Source: CAD feature listing. Evaluate the final solid. Frame: model axes, mm. Coordinates: 2 decimals unless noted, no trailing zeros. Loops run counter-clockwise (first coordinate to the right, second up) from the corner with the lowest first, then second, coordinate; pieces in that order, holes last.
```python
from build123d import *

# Parameters (mm, degrees)
SKETCH_1_R          = 2
SKETCH_1_R_2        = 11
EXTRUDE_1_DEPTH     = 4
SKETCH_3_W          = 126
SKETCH_3_H          = 2.7
CUT_EXTRUDE_1_DEPTH = 10


with BuildPart() as part:
    # 草图1 → 凸台-拉伸1 (new body)
    with BuildSketch(Plane.XY):
        Polygon((145, 46.5), (149, 46.5), (149, 45.15), (151.6, 45.15), (151.6, 46.5), (153.6, 46.5), (153.6, 49.5), (151.6, 49.5), (151.6, 50.85), (149, 50.85), (149, 49.5), (145, 49.5), (145, 59), (141, 59), (141, 67), (145, 67), (145, 76.5), (149, 76.5), (149, 75.15), (151.6, 75.15), (151.6, 76.5), (153.6, 76.5), (153.6, 79.5), (151.6, 79.5), (151.6, 80.85), (149, 80.85), (149, 79.5), (145, 79.5), (145, 89), (141, 89), (141, 97), (145, 97), (145, 106.5), (149, 106.5), (149, 105.15), (151.6, 105.15), (151.6, 106.5), (153.6, 106.5), (153.6, 109.5), (151.6, 109.5), (151.6, 110.85), (149, 110.85), (149, 109.5), (145, 109.5), (145, 123), (271, 123), (271, 109.5), (267, 109.5), (267, 110.85), (264.4, 110.85), (264.4, 109.5), (262.4, 109.5), (262.4, 106.5), (264.4, 106.5), (264.4, 105.15), (267, 105.15), (267, 106.5), (271, 106.5), (271, 97), (275, 97), (275, 89), (271, 89), (271, 79.5), (267, 79.5), (267, 80.85), (264.4, 80.85), (264.4, 79.5), (262.4, 79.5), (262.4, 76.5), (264.4, 76.5), (264.4, 75.15), (267, 75.15), (267, 76.5), (271, 76.5), (271, 67), (275, 67), (275, 59), (271, 59), (271, 49.5), (267, 49.5), (267, 50.85), (264.4, 50.85), (264.4, 49.5), (262.4, 49.5), (262.4, 46.5), (264.4, 46.5), (264.4, 45.15), (267, 45.15), (267, 46.5), (271, 46.5), (271, 37), (275, 37), (275, 29), (271, 29), (271, 19.5), (267, 19.5), (267, 20.85), (264.4, 20.85), (264.4, 19.5), (262.4, 19.5), (262.4, 16.5), (264.4, 16.5), (264.4, 15.15), (267, 15.15), (267, 16.5), (271, 16.5), (271, 7), (275, 7), (275, -1), (271, -1), (271, -10.5), (267, -10.5), (267, -9.15), (264.4, -9.15), (264.4, -10.5), (262.4, -10.5), (262.4, -13.5), (264.4, -13.5), (264.4, -14.85), (267, -14.85), (267, -13.5), (271, -13.5), (271, -27), (271, -34), (145, -34), (145, -27), (145, -13.5), (149, -13.5), (149, -14.85), (151.6, -14.85), (151.6, -13.5), (153.6, -13.5), (153.6, -10.5), (151.6, -10.5), (151.6, -9.15), (149, -9.15), (149, -10.5), (145, -10.5), (145, -1), (141, -1), (141, 7), (145, 7), (145, 16.5), (149, 16.5), (149, 15.15), (151.6, 15.15), (151.6, 16.5), (153.6, 16.5), (153.6, 19.5), (151.6, 19.5), (151.6, 20.85), (149, 20.85), (149, 19.5), (145, 19.5), (145, 29), (141, 29), (141, 37), (145, 37), align=None)
        with Locations((208, 29)):
            Circle(SKETCH_1_R, mode=Mode.SUBTRACT)
        with Locations((208, 48)):
            Circle(SKETCH_1_R_2, mode=Mode.SUBTRACT)
        with Locations((188, 8)):
            Circle(SKETCH_1_R, mode=Mode.SUBTRACT)
        with Locations((228, 8)):
            Circle(SKETCH_1_R, mode=Mode.SUBTRACT)
        with Locations((228, 88)):
            Circle(SKETCH_1_R, mode=Mode.SUBTRACT)
        with Locations((188, 88)):
            Circle(SKETCH_1_R, mode=Mode.SUBTRACT)
        with Locations((208, 8)):
            Circle(SKETCH_1_R, mode=Mode.SUBTRACT)
        with Locations((194.564971157, 34.564971157)):
            Circle(SKETCH_1_R, mode=Mode.SUBTRACT)
        with Locations((189, 48)):
            Circle(SKETCH_1_R, mode=Mode.SUBTRACT)
        with Locations((194.564971157, 61.435028843)):
            Circle(SKETCH_1_R, mode=Mode.SUBTRACT)
        with Locations((208, 67)):
            Circle(SKETCH_1_R, mode=Mode.SUBTRACT)
        with Locations((221.435028843, 61.435028843)):
            Circle(SKETCH_1_R, mode=Mode.SUBTRACT)
        with Locations((227, 48)):
            Circle(SKETCH_1_R, mode=Mode.SUBTRACT)
        with Locations((221.435028843, 34.564971157)):
            Circle(SKETCH_1_R, mode=Mode.SUBTRACT)
    extrude(amount=EXTRUDE_1_DEPTH)

    # 草图3 → 切除-拉伸1 (cut)
    with BuildSketch(Plane.XY.offset(4)):
        with Locations((208, 121.65)):
            Rectangle(SKETCH_3_W, SKETCH_3_H)
    extrude(amount=-CUT_EXTRUDE_1_DEPTH, mode=Mode.SUBTRACT)


solid = part.part
```
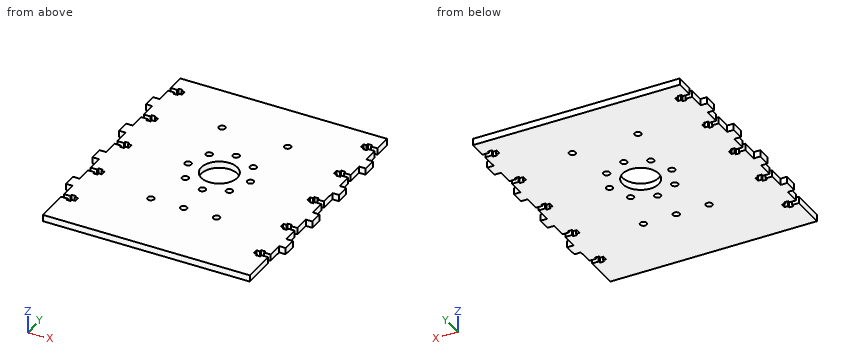
Q1. Material intervals for line 1 along Y through (x, z) = (149.5, 2); line 2 along Y through (x, z) = (269, 3.35); line 3 along Y through (x, z) = (208, 1.65), sorted ascending.
Q2. Section query B-B on z = 2.55. Count the separate pieces of the cut face and the enclosed holes in it, then the cut area to 3 significant figures.
Q3. First-contact query: pin 1 Ø1.1 at (y, z) = (-14, 2.5) entering from +X; pin 2 Ø1.1 at (y, z) = (105.5, 2.5) entering from -X; pin 3 Ø3 at (x, y) = (221.44, 34.56) entering from +Z; pin 4 Ø1.5 at (y, z) = (107.5, 2) entering from -X. Flat tips, straight axial feed; report the tip coordinate or a pass-through.
Q4. Section query A-A on x = 208. Return the cut outline in (y, z), then the cut area to 3 significant figures.
Resolved:
1. line 1: y = -34 to -14.85, -9.15 to 15.15, 20.85 to 45.15, 50.85 to 75.15, 80.85 to 105.15, 110.85 to 120.3
1. line 2: y = -34 to -13.5, -10.5 to 16.5, 19.5 to 46.5, 49.5 to 76.5, 79.5 to 106.5, 109.5 to 120.3
1. line 3: y = -34 to 6, 10 to 27, 31 to 37, 59 to 65, 69 to 120.3
2. separate pieces: 1
2. enclosed holes: 14
2. area: 18,800 mm2
3. pin 1: stops at x = 271
3. pin 2: stops at x = 145
3. pin 3: passes through
3. pin 4: stops at x = 153.6
4. outline: (-34, 0) - (6, 0) - (6, 4) - (-34, 4) - close; (10, 0) - (27, 0) - (27, 4) - (10, 4) - close; (31, 0) - (37, 0) - (37, 4) - (31, 4) - close; (59, 0) - (65, 0) - (65, 4) - (59, 4) - close; (69, 0) - (120.3, 0) - (120.3, 4) - (69, 4) - close
4. area: 481 mm2
